The figure shows three views and two pictorial views of one solid part (mm, origin at its lowest corner). Answer the questions. A direction names the side the tool comes from. Give positions to 0.01 mm unless a question says otherwise; leave off trailing zeros. Order: outer loops, then holes, each group sorted by start corner. A loop starts at its lowest first (then second) coordinate and runs counter-clockwise, first axis right, second up. Notation, with made-up numbers: (85.5, 78) - (112.5, 78) arc R20 ccw to (112.5, 95) - close; hole circle Ø8 at (10, -11.75). An arc over 180 degrees is marked (long way). Return JSON: item names as keys, results as strings. Group by question number.
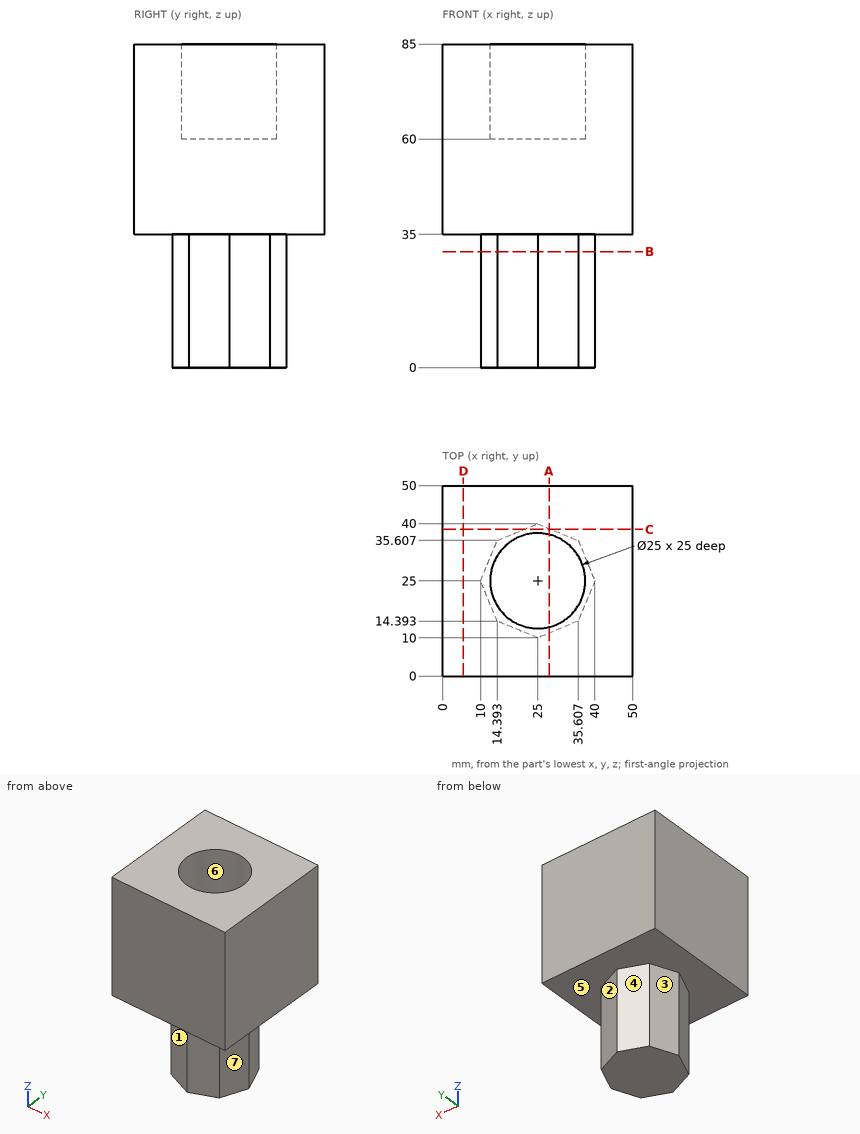
1. A tool of negligible diameter and unlimited length cuts with its end or side. For the marked faces 1, 2 and 3, from which of +Z, -Z, +X, -X, +Y, -Y can it reach the whole face along a straight path? Write none if from no direction.
2. Determine the mould class of the marked faces 4, 5, 6 and 7 for opening direction X: released by +X, released by -X, zero draft, split by the parting line, or undercut.
3. The part is cut by section D-D (x = 5.5). Give the vertices of the cut face in (y, z), and give its area (3 significant figures).
4. The part is cut by section B-B (z = 30.5). Give the vertices of the cut face in (x, y).
5. The part is cut by section A-A (x = 28). Give the vertices of the cut face in (y, z) (1 decimal), and give its area (3 significant figures).
6. Each of these flat-tipped pins is pushed along its axis until it touches: pin 1 (3 mm diameter, centred on y = 28.5, z = 26, fed in from -X); pin 2 (10 mm diameter, centred on y = 23, z = 9, fed in from -X). Where does it stop, or does it pass through?
7. Consider probe 1 along Y at (x, z) = (25, 67); probe 2 along Z at (x, y) = (5, 26); probe 3 along X at (y, z) = (18, 71) (1 decimal). Determine where each line is inside the solid, lowest interval first. Write a range as from..to.
8. The part is cut by section C-C (y = 38.5). Give the vertices of the cut face in (x, z).
Answers:
{
 "1": {"face 1": "-Z, -X, -Y", "face 2": "-Z, +X, +Y", "face 3": "-Z, -X, +Y"},
 "2": {"face 4": "released by -X", "face 5": "zero draft", "face 6": "undercut", "face 7": "released by +X"},
 "3": {"outline": "(0, 35) - (50, 35) - (50, 85) - (0, 85) - close", "area": "2,500 mm^2"},
 "4": {"outline": "(10, 25) - (14.39, 14.39) - (25, 10) - (35.61, 14.39) - (40, 25) - (35.61, 35.61) - (25, 40) - (14.39, 35.61) - close"},
 "5": {"outline": "(0, 35) - (11.2, 35) - (11.2, 0) - (38.8, 0) - (38.8, 35) - (50, 35) - (50, 85) - (37.1, 85) - (37.1, 60) - (12.9, 60) - (12.9, 85) - (0, 85) - close", "area": "2,860 mm^2"},
 "6": {"pin 1": "stops at x = 10.83", "pin 2": "stops at x = 10"},
 "7": {"probe 1": "y = 0..12.5, 37.5..50", "probe 2": "z = 35..85", "probe 3": "x = 0..14.6, 35.4..50"},
 "8": {"outline": "(0, 35) - (21.38, 35) - (21.38, 0) - (28.62, 0) - (28.62, 35) - (50, 35) - (50, 85) - (0, 85) - close"}
}
